Read the model definition and answer for the solid it produces. Units are mm, in the model's axes. Face numbers are marked on the shaded views. Round coordinates to 2 decimals unless told otherwise and drop trailing zeros. Loops run counter-clockwise (first coordinate to the right, second up) from the corner with the lowest first, then second, coordinate; pieces in that order, holes last. Notation, with made-up numbers: M 24,35 L 35,35 A21 ccw 35,62 Z; hole C 76,56 d7. An arc over 180 degrees is marked long. Answer as CSV lines item,"result".
```python
from build123d import *

# Parameters (mm, degrees)
F0_R     = 63.6619772368
F0_R_2   = 57.15
F1_DEPTH = 3
F2_R     = 67.15
F2_R_2   = 63.6619772368
F3_DEPTH = 5
F4_R     = 67.15
F4_R_2   = 63.6619772368
F4_R_3   = 57.15
F5_DEPTH = 5


with BuildPart() as f1:
    # F0 (on Top) → F1 (new body)
    with BuildSketch(Plane.XY):
        Circle(F0_R)
        Circle(F0_R_2, mode=Mode.SUBTRACT)
    extrude(amount=F1_DEPTH)

    # F2 (on face) + F0 (on Top) → F3 (join)
    with BuildSketch(Plane.XY):
        Circle(F2_R)
        Circle(F2_R_2, mode=Mode.SUBTRACT)
    with BuildSketch(Plane.XY):
        Circle(F0_R)
        Circle(F0_R_2, mode=Mode.SUBTRACT)
    extrude(amount=-F3_DEPTH)

    # F4 (on face) → F5 (join)
    with BuildSketch(Plane.XY.offset(3)):
        Circle(F4_R)
        Circle(F4_R_2, mode=Mode.SUBTRACT)
        Circle(F4_R_2)
        Circle(F4_R_3, mode=Mode.SUBTRACT)
    extrude(amount=F5_DEPTH)


solid = f1.part
```
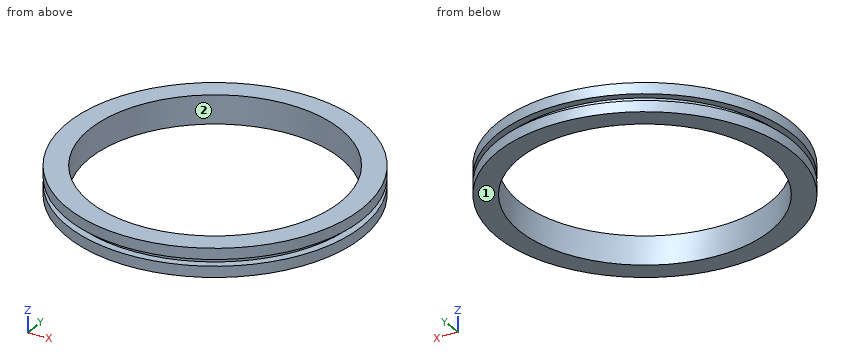
1) Determine the mould class of the marked faces 1 and 2 for opening direction Y: released by +Y, released by -Y, zero draft, split by the parting line, or undercut.
Evaluation:
face 1,"zero draft"
face 2,"undercut"
2) Find section C-C, the plane z = -2.5. Give the vertices of the cut face in (x, y).
Evaluation:
outline,"C 0,0 d134.3; hole C 0,0 d114.3"
3) Each of these flat-tipped pins is pushed along its axis until it touches: P1, Ø1, axis at y = 38, z = -1.5, coming from the -X side; P2, Ø1, axis at x = -2.5, z = -1, coming from the -Y side; P3, Ø6, axis at x = -52.5, z = -3, coming from the -Y side. Where does it stop, or does it pass through?
Evaluation:
P1,"stops at x = -55.7"
P2,"stops at y = -67.12"
P3,"stops at y = -45.37"
4) Straight lines are drawn through the part: line 1 (Z direction, x = -20, y = -61); line 2 (Y direction, x = 0, z = -2.25); line 3 (Y direction, x = 0, z = 2.75). For each, find the intervals that lie inside material, in ascending order.
Evaluation:
line 1,"z = -5 to 0, 3 to 8"
line 2,"y = -67.15 to -57.15, 57.15 to 67.15"
line 3,"y = -63.66 to -57.15, 57.15 to 63.66"
5) Find section A-A, the plane y = 0. Give the vertices of the cut face in (x, z), then the cut area to 3 significant figures.
Evaluation:
outline,"M -67.15,-5 L -57.15,-5 L -57.15,8 L -67.15,8 L -67.15,3 L -63.66,3 L -63.66,0 L -67.15,0 Z; M 57.15,-5 L 67.15,-5 L 67.15,0 L 63.66,0 L 63.66,3 L 67.15,3 L 67.15,8 L 57.15,8 Z"
area,"239 mm^2"
